Source: CAD feature listing. Evaluate the final solid. Frame: model axes, mm. A direction names the side the tool comes from. Give positions to 0.01 mm unless a question says otherwise; leave off trailing zeros. Loops run counter-clockwise (first coordinate to the right, second up) from the corner with the lowest first, then second, coordinate; pieces in that order, holes last.
```python
from build123d import *

# Parameters (mm, degrees)
SKETCH1_W           = 76.2
SKETCH1_H           = 25.4
SKETCH1_W_2         = 69.85
SKETCH1_H_2         = 19.05
EXTRUDE_THIN1_DEPTH = 146.05
CUT_EXTRUDE7_DEPTH  = 26.4
SKETCH7_R           = 3.175
CUT_EXTRUDE8_DEPTH  = 77.2
SKETCH8_R           = 2.4892
CUT_EXTRUDE9_DEPTH  = 77.2


with BuildPart() as part:
    # Sketch1 → Extrude-Thin1 (new body)
    with BuildSketch(Plane.XY):
        Rectangle(SKETCH1_W, SKETCH1_H)
        Rectangle(SKETCH1_W_2, SKETCH1_H_2, mode=Mode.SUBTRACT)
    extrude(amount=EXTRUDE_THIN1_DEPTH)

    # Sketch6 → Cut-Extrude7 (cut, through all)
    with BuildSketch(Plane(origin=(0, 12.7, 0), x_dir=(1, 0, 0), z_dir=(0, 1, 0))):
        with BuildLine():
            Line((-38.1, 0), (-38.1, -12.7))
            Line((-38.1, -12.7), (-25.4, -12.7))
            Line((-25.4, -12.7), (-25.4, -47.004160739))
            ThreePointArc((-25.4, -47.004160739), (-23.071797148, -50.064154136), (-19.501694746, -48.636408727))
            ThreePointArc((-19.501694746, -48.636408727), (0, -37.588701622), (19.501694746, -48.636408727))
            ThreePointArc((19.501694746, -48.636408727), (23.071797148, -50.064154136), (25.4, -47.004160739))
            Line((25.4, -47.004160739), (25.4, -12.7))
            Line((25.4, -12.7), (38.1, -12.7))
            Line((38.1, -12.7), (38.1, 0))
            Line((38.1, 0), (-38.1, 0))
        make_face()
    cut_extrude7 = extrude(amount=-CUT_EXTRUDE7_DEPTH, mode=Mode.SUBTRACT)

    # Sketch7 → Cut-Extrude8 (cut, through all)
    with BuildSketch(Plane(origin=(38.1, 0, 0), x_dir=(0, 0, -1), z_dir=(1, 0, 0))):
        with Locations((-27.686, 0)):
            Circle(SKETCH7_R)
    cut_extrude8 = extrude(amount=-CUT_EXTRUDE8_DEPTH, mode=Mode.SUBTRACT)

    # Mirror3: Cut-Extrude7, Cut-Extrude8 across plane
    add(cut_extrude7.mirror(Plane.XY.offset(73.025)), mode=Mode.SUBTRACT)
    add(cut_extrude8.mirror(Plane.XY.offset(73.025)), mode=Mode.SUBTRACT)

    # Sketch8 → Cut-Extrude9 (cut, through all)
    with BuildSketch(Plane.ZY.offset(38.1)):
        with Locations((46.736, 0)):
            Circle(SKETCH8_R)
        with Locations((99.314, 0)):
            Circle(SKETCH8_R)
        with Locations((80.264, 0)):
            Circle(SKETCH8_R)
        with Locations((65.786, 0)):
            Circle(SKETCH8_R)
    extrude(amount=-CUT_EXTRUDE9_DEPTH, mode=Mode.SUBTRACT)


solid = part.part
```
(1) Reachability of faces 4 (the flat face through (-1, -12.7, 72)), 5 (the flat face through (-25.4, -11, 30)), 6 (the flat face through (-25.4, -11, 116)), 7 (the flat face through (-34.925, 0, 72)) from +Z, -Z, +X, -X, +Y, -Y: full face, straight path, thin tool, end or side. Return the list, or none.
A:
face 4: +Z, -Z, +X, -X, -Y
face 5: -Z, +Y, -Y
face 6: +Z, +Y, -Y
face 7: +Z, -Z
(2) Section D-D, the plane z = 55.5. Return the cut outline in (x, y) (3 decimals), then the cut area to 3 significant figures.
A:
outline: (-38.1, -12.7) - (38.1, -12.7) - (38.1, 12.7) - (-38.1, 12.7) - close; hole (-34.925, -9.525) - (34.925, -9.525) - (34.925, 9.525) - (-34.925, 9.525) - close
area: 605 mm2
(3) First-contact query: pin 1 (1.5 mm diameter, centred on x = -19.5, y = -9.5, fed in from -Z); pin 2 (2 mm diameter, centred on x = 20, y = -10, fed in from +Z). Flat tips, straight axial feed; report the tip coordinate or a pass-through.
A:
pin 1: stops at z = 47.47
pin 2: stops at z = 98.21
(4) Mould query, pull axis X, two halves, no side actions, for faces 1 (the cylindrical face through (-36.535, 0.109, 77.777)), 2 (the flat face through (38.1, 0, 72)), 3 (the cylindrical face through (-23.127, -11.09, 50.048)). Classes: pulls with the +X half, pulls with the -X half, needs draft (parallel to the pull), parting line crosses it, or undercut.
A:
face 1: needs draft
face 2: pulls with the +X half
face 3: undercut
(5) Section A-A, the plane y = 5.5. Return the cut outline in (x, z) (3 decimals).
A:
outline: (-38.1, 12.7) - (-34.925, 12.7) - (-34.925, 133.35) - (-38.1, 133.35) - close; (34.925, 12.7) - (38.1, 12.7) - (38.1, 133.35) - (34.925, 133.35) - close
(6) Ray query, line 1 along Y through (x, z) = (13.5, 74) (3 decimals); line 2 along X through (y, z) = (8, 107) (3 decimals); line 3 along Z through (x, y) = (10.5, -11). Return the intervals inside material, ascending.
A:
line 1: y = -12.7 to -9.525, 9.525 to 12.7
line 2: x = -38.1 to -34.925, 34.925 to 38.1
line 3: z = 40.16 to 105.89
(7) Section C-C, the plane x = 29.5. Return the cut outline in (y, z) (3 decimals).
A:
outline: (-12.7, 12.7) - (-9.525, 12.7) - (-9.525, 133.35) - (-12.7, 133.35) - close; (9.525, 12.7) - (12.7, 12.7) - (12.7, 133.35) - (9.525, 133.35) - close
(8) Section B-B, the plane z = 35.5. Return the cut outline in (x, y) (3 decimals).
A:
outline: (-38.1, -12.7) - (-25.4, -12.7) - (-25.4, -9.525) - (-34.925, -9.525) - (-34.925, 9.525) - (-25.4, 9.525) - (-25.4, 12.7) - (-38.1, 12.7) - close; (25.4, -12.7) - (38.1, -12.7) - (38.1, 12.7) - (25.4, 12.7) - (25.4, 9.525) - (34.925, 9.525) - (34.925, -9.525) - (25.4, -9.525) - close
